The listing builds one solid part. Answer for the finished solid, in the listing's coordinates (mm). Round coordinates to 2 decimals unless told otherwise and drop trailing zeros. Loops run counter-clockwise (first coordinate to the right, second up) from the corner with the lowest first, then second, coordinate; pieces in that order, holes last. Notation, with made-up numbers: (59, 37) -> (109, 37) arc R7 ccw to (109, 50) -> close; hole circle Ø3 at (19.25, 63). An arc over 180 degrees is marked (long way). Use a Markdown table: item, result. Add a question column.
Q1. Section D-D on x = 40.5 is taken. Give the vertices of the cut face in (y, z).
Q2. Section B-B on x = -4 is taken. Give the vertices of the cut face in (y, z).
Q3. For a pull along X with two mould halves and no side action, classify faces 1 (the cylindrical face through (44.23, -25.27, 0.78)), 2 (the flat face through (-1, 1, 0)) as released by +X, released by -X, zero draft, split by the parting line, or undercut.
Q4. Consider line 1 (Y direction, x = 0, z = 1.25); line 2 (X direction, y = 14.5, z = 1.35) (3 decimals); line 3 (Y direction, x = -42, z = 0.8). Determine where each line is inside the solid, lowest interval first.
Q5. Section C-C on y = -24 is taken. Give the vertices of the cut face in (x, z) (1 decimal), then the cut area to 3 significant figures.
Q6. Section A-A on y = 19 is taken. Give the vertices of the cut face in (x, z) (1 decimal).
Q7. Given pin 1 Ø9 at (x, y) = (-41.783, -24.003) entering from -Z; pin 2 Ø0.8 at (x, z) = (-4, 0.5) entering from +Y; pin 3 Ø3.5 at (x, y) = (41.783, -24.003) entering from -Z, each flat-ended and moving along its own axis, determine where each tip first touches the part or whether it passes through.
Autodesk Inventor part; units mm, degrees
ref_plane "YZ Plane" through (0, 0, 0) normal (1, 0, 0) x (0, 1, 0)
ref_plane "XZ Plane" through (0, 0, 0) normal (0, 1, 0) x (-1, 0, 0)
ref_plane "XY Plane" through (0, 0, 0) normal (0, 0, 1) x (1, 0, 0)
sketch "Sketch1" plane through (0, 0, 0) normal (0, 0, 1) x (1, 0, 0)
  line L0 (0, -55.6514) -> (0, 55.6514)
  line L1 (52.705, 39.751) -> (52.705, -39.751)
  line L2 (52.705, -39.751) -> (-52.705, -39.751)
  line L3 (-52.705, -39.751) -> (-52.705, 39.751)
  line L4 (-73.787, 0) -> (73.787, 0)
  line L5 (-14.351, 39.751) -> (-14.351, 11.049)
  line L6 (-14.351, 11.049) -> (14.351, 11.049)
  line L7 (14.351, 11.049) -> (14.351, 39.751)
  line L8 (-52.705, 39.751) -> (-14.351, 39.751)
  line L9 (14.351, 39.751) -> (52.705, 39.751)
  line L10 (0, -39.751) -> (0, -14.097)
  circle A0 centre (0, -14.097) radius 14.2875
  point P0 (0, 0)
  dimension "d0" = 105.41
  dimension "d1" = 79.502
  dimension "d2" = 28.702
  dimension "d3" = 28.702
  dimension "d4" = 25.654
  dimension "d5" = 28.575
extrude "Extrusion1" add sketch "Sketch1" along normal blind 1.5875 contours L2 L3 L4 A0 L0 | L0 A0 L4 L1 L2 | L4 L3 L8 L5 L6 L0 A0 | L4 A0 L0 L6 L7 L9 L1
sketch "Sketch2" plane through (0, 0, 1.5875) normal (0, 0, 1) x (1, 0, 0)
  line L0 (52.705, -39.751) -> (52.705, 39.751)
  line L1 (-52.705, -39.751) -> (52.705, -39.751)
  point P0 (0, 0)
  point P1 (41.783, 24.257)
  point P2 (41.783, -24.003)
  dimension "d15" = 48.26
  dimension "d16" = 10.922
  dimension "d17" = 10.922
  dimension "d18" = 15.748
hole "Hole1" at (41.783, 24.257, 1.5875) at (41.783, -24.003, 1.5875) direction (0, 0, -1) diameter 5.5118 end through all
mirror "Mirror1" about plane through (0, 0, 0) normal (1, 0, 0) of "Hole1"
properties part number "DIFF_ROD"
Checked values:
| question | item | result |
|---|---|---|
| 1 | outline | (-39.75, 0) -> (-26.44, 0) -> (-26.44, 1.59) -> (-39.75, 1.59) -> close; (-21.56, 0) -> (21.82, 0) -> (21.82, 1.59) -> (-21.56, 1.59) -> close; (26.7, 0) -> (39.75, 0) -> (39.75, 1.59) -> (26.7, 1.59) -> close |
| 2 | outline | (-39.75, 0) -> (-27.81, 0) -> (-27.81, 1.59) -> (-39.75, 1.59) -> close; (-0.38, 0) -> (11.05, 0) -> (11.05, 1.59) -> (-0.38, 1.59) -> close |
| 3 | face 1 | undercut |
| 3 | face 2 | zero draft |
| 4 | line 1 | y = -39.75 to -28.38, 0.19 to 11.05 |
| 4 | line 2 | x = -52.705 to -14.351, 14.351 to 52.705 |
| 4 | line 3 | y = -39.75 to -26.75, -21.26 to 21.51, 27 to 39.75 |
| 5 | outline | (-52.7, 0) -> (-44.5, 0) -> (-44.5, 1.6) -> (-52.7, 1.6) -> close; (-39, 0) -> (-10.3, 0) -> (-10.3, 1.6) -> (-39, 1.6) -> close; (10.3, 0) -> (39, 0) -> (39, 1.6) -> (10.3, 1.6) -> close; (44.5, 0) -> (52.7, 0) -> (52.7, 1.6) -> (44.5, 1.6) -> close |
| 5 | area | 117 mm2 |
| 6 | outline | (-52.7, 0) -> (-14.4, 0) -> (-14.4, 1.6) -> (-52.7, 1.6) -> close; (14.4, 0) -> (52.7, 0) -> (52.7, 1.6) -> (14.4, 1.6) -> close |
| 7 | pin 1 | stops at z = 0 |
| 7 | pin 2 | stops at y = 11.05 |
| 7 | pin 3 | passes through |
